For this review, take the finished solid that the model builds, in its own axes (mm). A direction names the side the tool comes from. Round coordinates to 2 decimals unless told otherwise and drop trailing zeros. Order: outer loops, then holes, each group sorted by start corner. A loop starts at its lowest first (then second) coordinate and runs counter-clockwise, first axis right, second up. Notation, with made-up numbers: (86.25, 31) - (122.25, 31) arc R22 ccw to (122.25, 43) - close; hole circle Ø3 at (27, -37). An arc over 180 degrees is marked (long way). One line per item, written item: value.
```python
from build123d import *

# Parameters (mm, degrees)
SKETCH1_R           = 30
BOSS_EXTRUDE1_DEPTH = 250
SKETCH2_R           = 25
BOSS_EXTRUDE2_DEPTH = 15


with BuildPart() as part:
    # Sketch1 → Boss-Extrude1 (new body)
    with BuildSketch(Plane(origin=(0, 0, 0), x_dir=(0, 0, -1), z_dir=(1, 0, 0))):
        Circle(SKETCH1_R)
    extrude(amount=BOSS_EXTRUDE1_DEPTH)

    # Sketch2 → Boss-Extrude2 (add)
    with BuildSketch(Plane(origin=(250, 0, 0), x_dir=(0, 0, -1), z_dir=(1, 0, 0))):
        Circle(SKETCH2_R)
    extrude(amount=BOSS_EXTRUDE2_DEPTH)

    # Sketch3 → Revolve1 (revolve)
    with BuildSketch(Plane.XY):
        with BuildLine():
            Line((0, 30), (0, 0))
            Line((0, 0), (-250, 0))
            add(Edge.make_bspline(
                [(-250, 0), (-221.595628815, 6.156403899), (-140.370037823, 29.832530631), (-54.498709962, 27.773824359), (0, 30)],
                knots=[0, 0, 0, 0, 0.345336629, 1, 1, 1, 1], degree=3))
        make_face()
    revolve(axis=Axis((0, 0, 0), (-1, 0, 0)))


solid = part.part
```
Item 1: Machinability: for faces 1 (the flat face through (265, 0, 0)), 2 (the cylindrical face through (257.395, 7.509, -23.846)), which of the approach directions +Z, -Z, +X, -X, +Y, -Y give a long, thin tool a straight path to every point of the face, cutting with its end or side? Answer none if there is none.
Returned:
face 1: +Z, -Z, +X, +Y, -Y
face 2: +X
Item 2: Wall thickness on line 1 (Y direction, x = 11, z = 11); line 2 (Y direction, x = 106, z = -15); line 3 (Z direction, x = -132.5, y = -0.5): over which ranges is each line inside the solid? List them lowest first.
Returned:
line 1: -27.91 to 27.91
line 2: -25.98 to 25.98
line 3: -24 to 24
Item 3: Take a section at A-A (x = 28). Write out the cut boundary in (y, z), plus the area to 3 significant figures.
Returned:
outline: circle Ø60 at (0, 0)
area: 2,830 mm^2
Item 4: For P1, Ø12, axis at x = -2.5, y = 7.5, coming from the +Z side; P2, Ø4, axis at x = 75.5, y = 19, coming from the +Z side; P3, Ø4, axis at x = 132, z = 21.5, coming from the +Y side, all flat-tipped, find the tip position at first contact; note any pin that passes through.
Returned:
P1: z = 29.93
P2: z = 24.72
P3: y = 22.8
